```python
from build123d import *

# Parameters (mm, degrees)
EXTRUDE_1_DEPTH     = 15
SKETCH_2_R          = 1.6
SKETCH_2_R_2        = 6.25
CUT_EXTRUDE_1_DEPTH = 2
SKETCH_3_R          = 1.35
CUT_EXTRUDE_2_DEPTH = 31.5
FILLET_1_R          = 2


with BuildPart() as part:
    # 草图1 → 凸台-拉伸1 (new, symmetric)
    with BuildSketch(Plane(origin=(0, 0, 0), x_dir=(1, 0, 0), z_dir=(0, 1, 0))):
        with BuildLine():
            Line((0, 0), (22, 0))
            ThreePointArc((22, 0), (24.828427125, 1.171572875), (26, 4))
            Line((26, 4), (26, 26.5))
            Line((26, 26.5), (24, 26.5))
            Line((24, 26.5), (24, 4))
            ThreePointArc((24, 4), (23.414213562, 2.585786438), (22, 2))
            Line((22, 2), (0, 2))
            Line((0, 2), (-22, 2))
            ThreePointArc((-22, 2), (-23.414213562, 2.585786438), (-24, 4))
            Line((-24, 4), (-24, 26.5))
            Line((-24, 26.5), (-26, 26.5))
            Line((-26, 26.5), (-26, 4))
            ThreePointArc((-26, 4), (-24.828427125, 1.171572875), (-22, 0))
            Line((-22, 0), (0, 0))
        make_face()
    extrude(amount=EXTRUDE_1_DEPTH, both=True)

    # 草图2 → 切除-拉伸1 (cut)
    with BuildSketch(Plane(origin=(0, 0, -2), x_dir=(-1, 0, 0), z_dir=(0, 0, -1))):
        with Locations((20, 10.5)):
            Circle(SKETCH_2_R)
        with Locations((8.5, 8.5)):
            Circle(SKETCH_2_R)
        with Locations((-8.5, 8.5)):
            Circle(SKETCH_2_R)
        with Locations((-20, 10.5)):
            Circle(SKETCH_2_R)
        with Locations((-20, -10.5)):
            Circle(SKETCH_2_R)
        with Locations((8.5, -8.5)):
            Circle(SKETCH_2_R)
        with Locations((-8.5, -8.5)):
            Circle(SKETCH_2_R)
        with Locations((20, -10.5)):
            Circle(SKETCH_2_R)
        Circle(SKETCH_2_R_2)
    extrude(amount=-CUT_EXTRUDE_1_DEPTH, mode=Mode.SUBTRACT)

    # 草图3 → 切除-拉伸2 (cut, symmetric)
    with BuildSketch(Plane(origin=(0, 0, 0), x_dir=(0, 0, -1), z_dir=(1, 0, 0))):
        with Locations((10.5, 12)):
            Circle(SKETCH_3_R)
        with Locations((22.5, 12)):
            Circle(SKETCH_3_R)
        with Locations((10.5, 0)):
            Circle(SKETCH_3_R)
        with Locations((22.5, -12)):
            Circle(SKETCH_3_R)
        with Locations((10.5, -12)):
            Circle(SKETCH_3_R)
        with BuildLine():
            Line((22.5, 6.25), (26.5, 6.25))
            Line((26.5, 6.25), (26.5, -6.25))
            Line((26.5, -6.25), (22.5, -6.25))
            ThreePointArc((22.5, -6.25), (16.25, 0), (22.5, 6.25))
        make_face()
    extrude(amount=CUT_EXTRUDE_2_DEPTH, both=True, mode=Mode.SUBTRACT)

    # 圆角1
    fillet_1_edges = [part.edges().sort_by_distance(p)[0] for p in [
        (-25, 6.25, -26.5),
        (25, 6.25, -26.5),
        (-25, -6.25, -26.5),
        (25, -6.25, -26.5),
        (25, -15, -26.5),
        (-25, -15, -26.5),
        (-25, 15, -26.5),
        (25, 15, -26.5),
    ]]
    fillet(fillet_1_edges, radius=FILLET_1_R)


solid = part.part
```
The listing builds one solid part. Answer for the finished solid, in the listing's coordinates (mm). A direction names the side the tool comes from. Coordinates: 2 decimals unless noted, no trailing zeros. Write each loop counter-clockwise with the first axis right and the second up, starting at its lowest first coordinate (ties: lowest second). Pieces come first, ordered by that corner, then holes. Notation, with made-up numbers: (59, -12) -> (88, -12) arc R30 ccw to (88, 26) -> close; hole circle Ø4 at (-16, 35.25). An arc over 180 degrees is marked (long way). Write each question's results on one line, items separated by ' | '. Start each with the question number.
1) A cutting plane is placed at A-A (z = -6.5). Determine the outline of the cut face in (x, y), then the cut area to 3 significant figures.
2) A cutting plane is placed at C-C (x = -20). Determine the outline of the cut face in (y, z).
3) A tool of negligible diameter and unlimited length cuts with its end or side. For faces 1 (the cylindrical face through (24.99, -6.85, -25.93)), 2 (the cylindrical face through (24.99, 14.43, -25.9)), from which of +Z, -Z, +X, -X, +Y, -Y can it reach the whole face along a straight path? Write none if from no direction.
4) Flat-ended cylindrical pins translate along their axes: pin 1 Ø10 at (x, z) = (-15, -3.5) entering from -Y; pin 2 Ø5 at (x, y) = (-8.5, -8.5) entering from -Z. Find the tip coordinate at first contact, or state that the pin passes through.
5) Straight lines are drawn through the part: probe 1 along Y at (x, z) = (-24.7, -10.5); probe 2 along Y at (x, z) = (24.85, -22.5); probe 3 along Y at (x, z) = (20, -0.9). For each, find the intervals that lie inside material, in ascending order.
6) A cutting plane is placed at B-B (y = 0). Determine the outline of the cut face in (x, z), then the cut area to 3 significant figures.
7) A cutting plane is placed at D-D (x = 0). Determine the outline of the cut face in (y, z), then the cut area to 3 significant figures.
8) For a pull along X with two mould halves and no side action, classify faces 3 (the cylindrical face through (-7.23, -9.47, -1.01)), 4 (the flat face through (26, 0, -15)), 5 (the cylindrical face through (-24.986, 13.138, -11.226)), 6 (the cylindrical face through (-18.73, -11.47, -1.01)) as +X half, -X half, draft (parallel to the pull), parting line (faces both ways), or undercut.
Values follow:
1) outline: (-26, -15) -> (-24, -15) -> (-24, 15) -> (-26, 15) -> close; (24, -15) -> (26, -15) -> (26, 15) -> (24, 15) -> close | area: 120 mm²
2) outline: (-15, -2) -> (-12.1, -2) -> (-12.1, 0) -> (-15, 0) -> close; (-8.9, -2) -> (8.9, -2) -> (8.9, 0) -> (-8.9, 0) -> close; (12.1, -2) -> (15, -2) -> (15, 0) -> (12.1, 0) -> close
3) face 1: -Z, +X, -X | face 2: -Z, +X, -X, +Y
4) pin 1: y = -15 | pin 2: z = -2
5) probe 1: -15 to -13.35, -10.65 to -1.35, 1.35 to 10.65, 13.35 to 15 | probe 2: -15 to -13.35, -10.65 to -6.25, 6.25 to 10.65, 13.35 to 15 | probe 3: -15 to -12.1, -8.9 to 8.9, 12.1 to 15
6) outline: (-26, -16.25) -> (-24, -16.25) -> (-24, -11.85) -> (-26, -11.85) -> close; (-26, -9.15) -> (-24, -9.15) -> (-24, -4) arc R2 cw to (-22, -2) -> (-6.25, -2) -> (-6.25, 0) -> (-22, 0) arc R4 ccw to (-26, -4) -> close; (6.25, -2) -> (22, -2) arc R2 cw to (24, -4) -> (24, -9.15) -> (26, -9.15) -> (26, -4) arc R4 ccw to (22, 0) -> (6.25, 0) -> close; (24, -16.25) -> (26, -16.25) -> (26, -11.85) -> (24, -11.85) -> close | area: 120 mm²
7) outline: (-15, -2) -> (-6.25, -2) -> (-6.25, 0) -> (-15, 0) -> close; (6.25, -2) -> (15, -2) -> (15, 0) -> (6.25, 0) -> close | area: 35.0 mm²
8) face 3: undercut | face 4: +X half | face 5: draft | face 6: undercut
